Here's how the part is built. I have some questions about the finished solid (model axes, mm). A direction names the side the tool comes from. Round coordinates to 2 decimals unless told otherwise and drop trailing zeros. Write each loop counter-clockwise with the first axis right and the second up, starting at its lowest first coordinate (ties: lowest second). Pieces come first, ordered by that corner, then holes. Notation, with made-up numbers: M 35,-24.75 L 93,-24.75 A28 ccw 93,-4.75 Z; hole C 60,26.5 d10. An arc over 180 degrees is marked long. Use a Markdown table: item, result. Add a question column.
```python
from build123d import *

# Parameters (mm, degrees)
F1_DEPTH = 15.875
F3_DEPTH = 76.201
F5_DEPTH = 31.751
F6_F1_R  = 1.27
F6_F2_R  = 1.27


with BuildPart() as f1:
    # F0 (on Front) → F1 (new body, symmetric)
    with BuildSketch(Plane.XZ):
        Polygon((-38.1, 19.05), (-38.1, 0), (38.1, 0), (-31.75, 12.3164396025), (-31.75, 19.05), align=None)
    extrude(amount=F1_DEPTH, both=True)

    # F2 (on face) → F3 (cut, through all)
    with BuildSketch(Plane(origin=(-38.1, 0, 0), x_dir=(0, -1, 0), z_dir=(-1, 0, 0))):
        with BuildLine():
            Line((-10.922, 0), (-10.922, 3.81))
            ThreePointArc((-10.922, 3.81), (-12.5728756711, 5.4608756711), (-14.2237513422, 3.81))
            Line((-14.2237513422, 3.81), (-14.2237513422, 0))
            Line((-14.2237513422, 0), (-10.922, 0))
        make_face()
        with BuildLine():
            Line((14.2237513422, 0), (14.2237513422, 3.81))
            ThreePointArc((14.2237513422, 3.81), (12.5728756711, 5.4608756711), (10.922, 3.81))
            Line((10.922, 3.81), (10.922, 0))
            Line((10.922, 0), (14.2237513422, 0))
        make_face()
    extrude(amount=-F3_DEPTH, mode=Mode.SUBTRACT)

    # F4 (on face) → F5 (cut, through all)
    with BuildSketch(Plane(origin=(0, 15.875, 0), x_dir=(-1, 0, 0), z_dir=(0, 1, 0))):
        with BuildLine():
            ThreePointArc((29.083, 0), (25.4, 3.683), (21.717, 0))
            Line((21.717, 0), (29.083, 0))
        make_face()
    extrude(amount=-F5_DEPTH, mode=Mode.SUBTRACT)

    # F6: fillet of radius 1.27 on 17 edges, made by hand

    # F6_f1
    f6_f1_edges = [f1.edges().sort_by_distance(p)[0] for p in [
        (-31.75, 0, 12.3164396025),
    ]]
    fillet(f6_f1_edges, radius=F6_F1_R)

    # F6_f2
    f6_f2_edges = [f1.edges().sort_by_distance(p)[0] for p in [
        (38.1, 0, 0),
        (38.1, 15.0493756711, 0),
        (38.1, -15.0493756711, 0),
        (-31.75, 0, 19.05),
        (-38.1, 0, 19.05),
        (-38.1, 15.0493756711, 0),
        (-38.1, 0, 0),
        (-33.5915, -15.875, 0),
        (8.1915, 15.875, 0),
        (-33.5915, 15.875, 0),
        (3.6997334072, -15.875, 6.0656951439),
        (-38.1, -15.875, 9.525),
        (-38.1, 15.875, 9.525),
        (-34.925, -15.875, 19.05),
        (-34.925, 15.875, 19.05),
        (3.6997334072, 15.875, 6.0656951439),
        (-31.4528764428, 15.875, 12.5657558698),
        (-31.4528764428, -15.875, 12.5657558698),
    ]]
    fillet(f6_f2_edges, radius=F6_F2_R)


solid = f1.part
```
Item 1: Imagine slicing it at C-C on x = 15. Count the separate pieces of the cut face and the enclosed holes in it, plus the area to 3 significant figures.
Item 2: I need wall thicknesses on probe 1 along Y at (x, z) = (15, 2.25) (3 decimals); probe 2 along Y at (x, z) = (-18.5, 4.5) (3 decimals); probe 3 along X at (y, z) = (3, 16.75). Which ranges of each line are inside material? Lowest first, please. Write a range as from..to.
Item 3: Imagine slicing it at B-B on z = 15.25. List the corners of the cut face in (x, y) for me (3 decimals).
Item 4: Imagine slicing it at D-D on y = -13.5. List the corners of the cut face in (x, z) for me, plus the area to 3 significant figures.
Item 5: Imagine slicing it at A-A on y = -2.5. List the corners of the cut face in (x, z) for me.
Item 6: If we mould it in two halves opening along Y, with no side actions, what happens to faces 1 (the face through (-7, 10.922, 2)), 2 (the face through (24.85, 14.41, 1.19)), 3 (the face through (-18, 15.875, 6))? For each: +Y half, -Y half, draft (parallel to the pull), parting line (faces both ways), or undercut.
Item 7: On a 3-axis mill with a long thin cutter (end or side, diameter ignored), from which of +Z, -Z, +X, -X, +Y, -Y can I reach the whole of each face in a straight line? I mean faces 4 (the face through (-37.738, 14.412, 0.382)), 5 (the face through (-31.75, 0, 16)), 6 (the face through (-11.19, 12.54, 5.46)). Say none if no direction works.
Item 8: For pin 1 Ø3.5 at (y, z) = (0.5, 15) entering from +X; pin 2 Ø1 at (x, z) = (-2, 6.5) entering from +Y; pin 3 Ø4 at (x, y) = (-10, -9) entering from +Z, each with a flat end and sliding along its axis, tell me the tip position at first contact or that it passes through.
The answers:
| question | item | result |
|---|---|---|
| 1 | separate pieces | 3 |
| 1 | enclosed holes | 0 |
| 1 | area | 101 mm² |
| 2 | probe 1 | -15.875..-14.224, -10.922..10.922, 14.224..15.875 |
| 2 | probe 2 | -15.875..-14.073, -11.073..11.073, 14.073..15.875 |
| 2 | probe 3 | -38.1..-31.75 |
| 3 | outline | M -38.1,-14.605 A1.27 ccw -36.83,-15.875 L -33.02,-15.875 A1.27 ccw -31.75,-14.605 L -31.75,14.605 A1.27 ccw -33.02,15.875 L -36.83,15.875 A1.27 ccw -38.1,14.605 Z |
| 4 | outline | M -38.1,5.18 L 8.75,5.18 L -30.7,12.13 A1.27 cw -31.75,13.38 L -31.75,17.78 A1.27 ccw -33.02,19.05 L -36.83,19.05 A1.27 ccw -38.1,17.78 Z |
| 4 | area | 232 mm² |
| 5 | outline | M -38.1,1.27 A1.27 ccw -36.83,0 L -29.08,0 A3.68 cw -21.72,0 L 23.58,0 A1.27 ccw 23.8,2.52 L -30.7,12.13 A1.27 cw -31.75,13.38 L -31.75,17.78 A1.27 ccw -33.02,19.05 L -36.83,19.05 A1.27 ccw -38.1,17.78 Z |
| 6 | face 1 | undercut |
| 6 | face 2 | draft |
| 6 | face 3 | +Y half |
| 7 | face 4 | -Z, -X, +Y |
| 7 | face 5 | +Z, +X, +Y, -Y |
| 7 | face 6 | -Z, +X, -X |
| 8 | pin 1 | x = -31.74 |
| 8 | pin 2 | y = 15.86 |
| 8 | pin 3 | z = 8.83 |
